Work out the finished part from the listing and answer in its coordinate system (mm). A direction names the side the tool comes from. Coordinates: 2 decimals unless noted, no trailing zeros. One line per question, with ' | ' between items.
```python
from build123d import *

# Parameters (mm, degrees)
F1_DEPTH = 25


# Not quite as in the source:
# - ends of sketch curves that miss each other by under 0.0002 mm in the source are joined


with BuildPart() as f1:
    # F0 (on Top) → F1 (new body, symmetric)
    with BuildSketch(Plane.XY):
        with BuildLine():
            ThreePointArc((2.803779, 4.0132), (2.9218403787, 3.9330028938), (2.8907965459, 3.7936962341))
            Line((2.8907965459, 3.7936962341), (1.0639298, 2.075561))
            ThreePointArc((1.0639298, 2.075561), (0.9835034993, 2.0244706276), (0.8899144, 2.0066))
            Line((0.8899144, 2.0066), (0.7493, 2.0066))
            ThreePointArc((0.7493, 2.0066), (0.5696948776, 1.9322051224), (0.4953, 1.7526))
            ThreePointArc((0.4953, 1.7526), (0.4209051224, 1.5729948776), (0.2413, 1.4986))
            Line((0.2413, 1.4986), (-0.2413, 1.4986))
            ThreePointArc((-0.2413, 1.4986), (-0.4209051224, 1.5729948776), (-0.4953, 1.7526))
            ThreePointArc((-0.4953, 1.7526), (-0.5696948776, 1.9322051224), (-0.7493, 2.0066))
            Line((-0.7493, 2.0066), (-0.8899144, 2.0066))
            ThreePointArc((-0.8899144, 2.0066), (-0.9835034993, 2.0244706276), (-1.0639233392, 2.0755678701))
            Line((-1.0639233392, 2.0755678701), (-2.8907994, 3.7936932))
            ThreePointArc((-2.8907994, 3.7936932), (-2.9218403787, 3.9330028938), (-2.803779, 4.0132))
            Line((-2.803779, 4.0132), (-1.7526, 4.0132))
            ThreePointArc((-1.7526, 4.0132), (-1.5729948776, 4.0875948776), (-1.4986, 4.2672))
            Line((-1.4986, 4.2672), (-1.4986, 4.7498))
            ThreePointArc((-1.4986, 4.7498), (-1.5729948776, 4.9294051224), (-1.7526, 5.0038))
            Line((-1.7526, 5.0038), (-4.7498, 5.0038))
            ThreePointArc((-4.7498, 5.0038), (-4.9294051224, 4.9294051224), (-5.0038, 4.7498))
            Line((-5.0038, 4.7498), (-5.0038, 1.7526))
            ThreePointArc((-5.0038, 1.7526), (-4.9294051224, 1.5729948776), (-4.7498, 1.4986))
            Line((-4.7498, 1.4986), (-4.2672, 1.4986))
            ThreePointArc((-4.2672, 1.4986), (-4.0875948776, 1.5729948776), (-4.0132, 1.7526))
            Line((-4.0132, 1.7526), (-4.0132, 2.803779))
            ThreePointArc((-4.0132, 2.803779), (-3.9330028938, 2.9218403787), (-3.7936962341, 2.8907965459))
            Line((-3.7936962341, 2.8907965459), (-2.075561, 1.0639298))
            ThreePointArc((-2.075561, 1.0639298), (-2.0244706276, 0.9835034993), (-2.0066, 0.8899144))
            Line((-2.0066, 0.8899144), (-2.0066, 0.7493))
            ThreePointArc((-2.0066, 0.7493), (-1.9322051224, 0.5696948776), (-1.7526, 0.4953))
            ThreePointArc((-1.7526, 0.4953), (-1.5729948776, 0.4209051224), (-1.4986, 0.2413))
            Line((-1.4986, 0.2413), (-1.4986, -0.2413))
            ThreePointArc((-1.4986, -0.2413), (-1.5729948776, -0.4209051224), (-1.7526, -0.4953))
            ThreePointArc((-1.7526, -0.4953), (-1.9322051224, -0.5696948776), (-2.0066, -0.7493))
            Line((-2.0066, -0.7493), (-2.0066, -0.8899144))
            ThreePointArc((-2.0066, -0.8899144), (-2.0244706276, -0.9835034993), (-2.0755678701, -1.0639233392))
            Line((-2.0755678701, -1.0639233392), (-3.7936932, -2.8907994))
            ThreePointArc((-3.7936932, -2.8907994), (-3.9330028938, -2.9218403787), (-4.0132, -2.803779))
            Line((-4.0132, -2.803779), (-4.0132, -1.7526))
            ThreePointArc((-4.0132, -1.7526), (-4.0875948776, -1.5729948776), (-4.2672, -1.4986))
            Line((-4.2672, -1.4986), (-4.7498, -1.4986))
            ThreePointArc((-4.7498, -1.4986), (-4.9294051224, -1.5729948776), (-5.0038, -1.7526))
            Line((-5.0038, -1.7526), (-5.0038, -4.7498))
            ThreePointArc((-5.0038, -4.7498), (-4.9294051224, -4.9294051224), (-4.7498, -5.0038))
            Line((-4.7498, -5.0038), (-1.7526, -5.0038))
            ThreePointArc((-1.7526, -5.0038), (-1.5729948776, -4.9294051224), (-1.4986, -4.7498))
            Line((-1.4986, -4.7498), (-1.4986, -4.2672))
            ThreePointArc((-1.4986, -4.2672), (-1.5729948776, -4.0875948776), (-1.7526, -4.0132))
            Line((-1.7526, -4.0132), (-2.803779, -4.0132))
            ThreePointArc((-2.803779, -4.0132), (-2.9218403787, -3.9330028938), (-2.8907965459, -3.7936962341))
            Line((-2.8907965459, -3.7936962341), (-1.0639298, -2.075561))
            ThreePointArc((-1.0639298, -2.075561), (-0.9835034993, -2.0244706276), (-0.8899144, -2.0066))
            Line((-0.8899144, -2.0066), (-0.7493, -2.0066))
            ThreePointArc((-0.7493, -2.0066), (-0.5696948776, -1.9322051224), (-0.4953, -1.7526))
            ThreePointArc((-0.4953, -1.7526), (-0.4209051224, -1.5729948776), (-0.2413, -1.4986))
            Line((-0.2413, -1.4986), (0.2413, -1.4986))
            ThreePointArc((0.2413, -1.4986), (0.4209051224, -1.5729948776), (0.4953, -1.7526))
            ThreePointArc((0.4953, -1.7526), (0.5696948776, -1.9322051224), (0.7493, -2.0066))
            Line((0.7493, -2.0066), (0.8899144, -2.0066))
            ThreePointArc((0.8899144, -2.0066), (0.9835034993, -2.0244706276), (1.0639233392, -2.0755678701))
            Line((1.0639233392, -2.0755678701), (2.8907994, -3.7936932))
            ThreePointArc((2.8907994, -3.7936932), (2.9218403787, -3.9330028938), (2.803779, -4.0132))
            Line((2.803779, -4.0132), (1.7526, -4.0132))
            ThreePointArc((1.7526, -4.0132), (1.5729948776, -4.0875948776), (1.4986, -4.2672))
            Line((1.4986, -4.2672), (1.4986, -4.7498))
            ThreePointArc((1.4986, -4.7498), (1.5729948776, -4.9294051224), (1.7526, -5.0038))
            Line((1.7526, -5.0038), (4.7498, -5.0038))
            ThreePointArc((4.7498, -5.0038), (4.9294051224, -4.9294051224), (5.0038, -4.7498))
            Line((5.0038, -4.7498), (5.0038, -1.7526))
            ThreePointArc((5.0038, -1.7526), (4.9294051224, -1.5729948776), (4.7498, -1.4986))
            Line((4.7498, -1.4986), (4.2672, -1.4986))
            ThreePointArc((4.2672, -1.4986), (4.0875948776, -1.5729948776), (4.0132, -1.7526))
            Line((4.0132, -1.7526), (4.0132, -2.803779))
            ThreePointArc((4.0132, -2.803779), (3.9330028938, -2.9218403787), (3.7936962341, -2.8907965459))
            Line((3.7936962341, -2.8907965459), (2.075561, -1.0639298))
            ThreePointArc((2.075561, -1.0639298), (2.0244706276, -0.9835034993), (2.0066, -0.8899144))
            Line((2.0066, -0.8899144), (2.0066, -0.7493))
            ThreePointArc((2.0066, -0.7493), (1.9322051224, -0.5696948776), (1.7526, -0.4953))
            ThreePointArc((1.7526, -0.4953), (1.5729948776, -0.4209051224), (1.4986, -0.2413))
            Line((1.4986, -0.2413), (1.4986, 0.2413))
            ThreePointArc((1.4986, 0.2413), (1.5729948776, 0.4209051224), (1.7526, 0.4953))
            ThreePointArc((1.7526, 0.4953), (1.9322051224, 0.5696948776), (2.0066, 0.7493))
            Line((2.0066, 0.7493), (2.0066, 0.8899144))
            ThreePointArc((2.0066, 0.8899144), (2.0244706276, 0.9835034993), (2.0755678701, 1.0639233392))
            Line((2.0755678701, 1.0639233392), (3.7936932, 2.8907994))
            ThreePointArc((3.7936932, 2.8907994), (3.9330028938, 2.9218403787), (4.0132, 2.803779))
            Line((4.0132, 2.803779), (4.0132, 1.7526))
            ThreePointArc((4.0132, 1.7526), (4.0875948776, 1.5729948776), (4.2672, 1.4986))
            Line((4.2672, 1.4986), (4.7498, 1.4986))
            ThreePointArc((4.7498, 1.4986), (4.9294051224, 1.5729948776), (5.0038, 1.7526))
            Line((5.0038, 1.7526), (5.0038, 4.7498))
            ThreePointArc((5.0038, 4.7498), (4.9294051224, 4.9294051224), (4.7498, 5.0038))
            Line((4.7498, 5.0038), (1.7526, 5.0038))
            ThreePointArc((1.7526, 5.0038), (1.5729948776, 4.9294051224), (1.4986, 4.7498))
            Line((1.4986, 4.7498), (1.4986, 4.2672))
            ThreePointArc((1.4986, 4.2672), (1.5729948776, 4.0875948776), (1.7526, 4.0132))
            Line((1.7526, 4.0132), (2.803779, 4.0132))
        make_face()
    extrude(amount=F1_DEPTH, both=True)


solid = f1.part
```
1) The mould has two halves that part along X. Classify faces 1 (the face through (0, 0, 25)), 2 (the face through (5.004, -3, 0)), 3 (the face through (-4.013, 2, 0)): released by +X, released by -X, zero draft, split by the parting line, or undercut.
Check values:
face 1: zero draft | face 2: released by +X | face 3: undercut
2) A flat-ended cylindrical pin translates along its axis: pin 1 (1 mm diameter, centred on y = 1.5, z = 8.5, fed in from -X). Find the tip coordinate at first contact, or state that the pin passes through.
Check values:
pin 1: stops at x = -5
3) Find the intervals of material crossed by line 1 along X through (y, z) = (1.75, -14); line 2 along Y through (x, z) = (4.5, -6), in increasing order.
Check values:
line 1: x = -5 to -4.01, -2.72 to -0.5, 0.5 to 2.72, 4.01 to 5 | line 2: y = -5 to -1.5, 1.5 to 5
4) For faces 4 (the face through (-3, 5.004, 0)), 5 (the face through (-2, 4.013, 0)), determine the directions among +Z, -Z, +X, -X, +Y, -Y from which every point of the face is accessible in a straight line to the end or side of a thin tool.
Check values:
face 4: +Z, -Z, +X, -X, +Y | face 5: +Z, -Z
